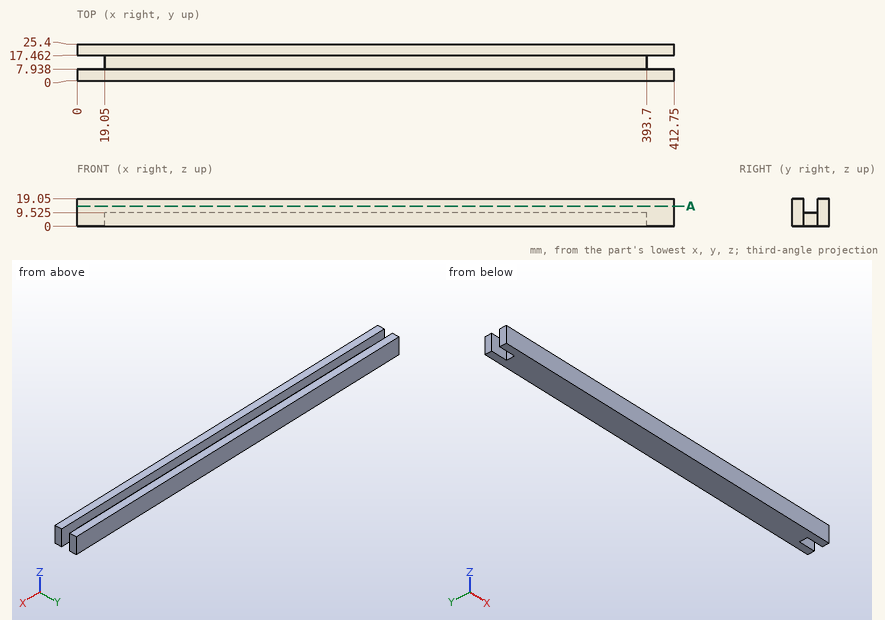
Design review of the part shown in the three views and the two pictorial views. Dimensions are in mm from the part's minimum x, y and z. Round coordinates to 2 decimals unless told otherwise and drop trailing zeros. Order: outer loops, then holes, each group sorted by start corner. A loop starts at its lowest first (then second) coordinate and runs counter-clockwise, first axis right, second up.
Item 1: To check wall thickness, follow probe 1 along Y at (x, z) = (123.5, 11.25); probe 2 along X at (y, z) = (11.25, 1.5); probe 3 along Z at (x, y) = (167.5, 11) (1 decimal). State the ranges of each line that lie inside material, in increasing order.
Working result:
probe 1: y = 0 to 7.94, 17.46 to 25.4
probe 2: x = 19.05 to 393.7
probe 3: z = 0 to 9.5
Item 2: Add section A-A, the plane z = 14. State the section outline as (x, y) points, and give its area (3 significant figures).
Working result:
outline: (0, 0) - (412.75, 0) - (412.75, 7.94) - (0, 7.94) - close; (0, 17.46) - (412.75, 17.46) - (412.75, 25.4) - (0, 25.4) - close
area: 6,550 mm2
Item 3: For pin 1 (5 mm diameter, centred on y = 12.5, z = 3.5, fed in from -X); pin 2 (4 mm diameter, centred on y = 10.5, z = 16.5, fed in from -X); pin 3 (2 mm diameter, centred on x = 278, y = 11, fed in from +Z) (1 decimal), all flat-tipped, find the tip position at first contact; note any pin that passes through.
Working result:
pin 1: stops at x = 19.05
pin 2: passes through
pin 3: stops at z = 9.5
